from build123d import *

# Parameters (mm, degrees)
SKETCH1_W           = 47
SKETCH1_H           = 38.8
SKETCH1_R           = 2.5
SKETCH1_R_2         = 2.627
BOSS_EXTRUDE1_DEPTH = 106.999989
SKETCH2_R           = 3.571875
SKETCH2_R_2         = 4.92125
CUT_EXTRUDE1_DEPTH  = 39.8
SKETCH1_8_R         = 2.627
SKETCH1_8_R_2       = 2.5
CUT_EXTRUDE2_DEPTH  = 38.1
CUT_EXTRUDE3_START  = -47
SKETCH3_R           = 2
CUT_EXTRUDE3_DEPTH  = 25.4
SKETCH4_R           = 9.525
CUT_EXTRUDE4_DEPTH  = 21.0185


with BuildPart() as part:
    # Sketch1 → Boss-Extrude1 (new body)
    with BuildSketch(Plane(origin=(0, 0, 0), x_dir=(1, 0, 0), z_dir=(0, 1, 0))):
        with Locations((23.5, 19.4)):
            Rectangle(SKETCH1_W, SKETCH1_H)
        with Locations((4.5, 4.4)):
            Circle(SKETCH1_R, mode=Mode.SUBTRACT)
        with Locations((42.5, 4.4)):
            Circle(SKETCH1_R, mode=Mode.SUBTRACT)
        with Locations((4.5, 34.4)):
            Circle(SKETCH1_R_2, mode=Mode.SUBTRACT)
        with Locations((42.5, 34.4)):
            Circle(SKETCH1_R, mode=Mode.SUBTRACT)
        with Locations((42.5, 4.4)):
            Circle(SKETCH1_R)
        with Locations((4.5, 4.4)):
            Circle(SKETCH1_R)
        with Locations((4.5, 34.4)):
            Circle(SKETCH1_R_2)
        with Locations((42.5, 34.4)):
            Circle(SKETCH1_R)
    extrude(amount=BOSS_EXTRUDE1_DEPTH)

    # Sketch2 → Cut-Extrude1 (cut, through all)
    with BuildSketch(Plane.XY):
        with Locations((12.36448241, 63.94291018)):
            Circle(SKETCH2_R)
        with Locations((34.63551759, 63.94291018)):
            Circle(SKETCH2_R)
        with Locations((34.63551759, 41.671875)):
            Circle(SKETCH2_R)
        with Locations((23.5, 52.80739259)):
            Circle(SKETCH2_R_2)
        with Locations((12.36448241, 41.671875)):
            Circle(SKETCH2_R)
    extrude(amount=-CUT_EXTRUDE1_DEPTH, mode=Mode.SUBTRACT)

    # Sketch1<8> → Cut-Extrude2 (cut)
    with BuildSketch(Plane(origin=(0, 0, 0), x_dir=(1, 0, 0), z_dir=(0, 1, 0))):
        with Locations((4.5, 34.4)):
            Circle(SKETCH1_8_R)
        with Locations((4.5, 4.4)):
            Circle(SKETCH1_8_R_2)
        with Locations((42.5, 4.4)):
            Circle(SKETCH1_8_R_2)
        with Locations((42.5, 34.4)):
            Circle(SKETCH1_8_R_2)
    extrude(amount=CUT_EXTRUDE2_DEPTH, mode=Mode.SUBTRACT)

    # Sketch3 → Cut-Extrude3 (cut)
    with BuildSketch(Plane(origin=(47, 0, 0), x_dir=(0, 0, -1), z_dir=(1, 0, 0)).offset(CUT_EXTRUDE3_START)):
        with Locations((19.4, 20)):
            Circle(SKETCH3_R)
        with Locations((19.4, 79.944)):
            Circle(SKETCH3_R)
    extrude(amount=CUT_EXTRUDE3_DEPTH, mode=Mode.SUBTRACT)

    # Sketch4 → Cut-Extrude4 (cut)
    with BuildSketch(Plane(origin=(0, 0, -38.8), x_dir=(-1, 0, 0), z_dir=(0, 0, -1))):
        with Locations((-23.5, 52.80739259)):
            Circle(SKETCH4_R)
    extrude(amount=-CUT_EXTRUDE4_DEPTH, mode=Mode.SUBTRACT)


solid = part.part
Verification items for the finished model (mm, model axes). A direction names the side the tool comes from. Coordinates: 2 decimals unless noted, no trailing zeros. Order: outer loops, then holes, each group sorted by start corner. A loop starts at its lowest first (then second) coordinate and runs counter-clockwise, first axis right, second up. Notation, with made-up numbers: (-22, 64) -> (-5, 64) arc R6 ccw to (-5, 68) -> close; hole circle Ø1 at (7.5, 55). An arc over 180 degrees is marked (long way). Put each result on its own line as item: value. Start each with the question number.
1. Cross-section at A-A, the plane x = 23.5. Record the boundary of the cut face in (y, z), then the cut area to 3 significant figures.
2. Cross-section at B-B, the plane y = 20. Record the boundary of the cut face in (x, z), then the cut area to 3 significant figures.
3. Access from +Z, -Z, +X, -X, +Y, -Y to the whole of each face (thin tool, end or side, straight path). Record for faces 1 (the flat face through (4, 38.1, -34)), 2 (the cylindrical face through (11.59, 60.456, -19.128)), 3 (the flat face through (25.4, 20, -19)).
4. Cross-section at C-C, the plane x = 12.5. Record the boundary of the cut face in (y, z), then the cut area to 3 significant figures.
5. Material ranges on L1, parallel to X at y = 13.5, z = -4.5; L2, parallel to Z at x = 42.5, y = 8.5; L3, parallel to X at y = 29, z = -34.4, recorded low to high. Write a range as [from, to].
6. Go/stop test with flat-tipped pins: pin 1 Ø15 at (x, y) = (23.5, 51) entering from -Z; pin 2 Ø4 at (x, z) = (4.5, -4.4) entering from -Y. Record where each tip stops, or that it passes through.
7. Cross-section at D-D, the plane z = -25. Record the boundary of the cut face in (x, y) (3 decimals), then the cut area to 3 significant figures.
8. Mould release check, pull along Z, two halves, no side actions. Record for faces 4 (the flat face through (18, 53, 0)), 5 (the flat face through (19, 49, -17.781)), 6 (the cylindrical face through (12.522, 20.601, -21.308)): released by +Z, released by -Z, zero draft, split by the parting line, or undercut.
Computed:
1. outline: (0, -38.8) -> (43.28, -38.8) -> (43.28, -17.78) -> (47.89, -17.78) -> (47.89, 0) -> (0, 0) -> close; (57.73, -17.78) -> (62.33, -17.78) -> (62.33, -38.8) -> (107, -38.8) -> (107, 0) -> (57.73, 0) -> close; hole circle Ø4 at (20, -19.4); hole circle Ø4 at (79.94, -19.4)
1. area: 3,550 mm2
2. outline: (0, -38.8) -> (47, -38.8) -> (47, 0) -> (0, 0) -> (0, -17.4) -> (25.4, -17.4) -> (25.4, -21.4) -> (0, -21.4) -> close; hole circle Ø5.25 at (4.5, -34.4); hole circle Ø5 at (4.5, -4.4); hole circle Ø5 at (42.5, -34.4); hole circle Ø5 at (42.5, -4.4)
2. area: 1,640 mm2
3. face 1: -Y
3. face 2: +Z, -Z
3. face 3: -X
4. outline: (0, -38.8) -> (38.1, -38.8) -> (38.1, 0) -> (0, 0) -> close; (45.24, -38.8) -> (60.37, -38.8) -> (60.37, 0) -> (45.24, 0) -> close; (67.51, -38.8) -> (107, -38.8) -> (107, 0) -> (67.51, 0) -> close; hole circle Ø4 at (20, -19.4); hole circle Ø4 at (79.94, -19.4)
4. area: 3,570 mm2
5. L1: [0, 2], [7, 40], [45, 47]
5. L2: [-38.8, -36.9], [-31.9, -6.9], [-1.9, 0]
5. L3: [0, 1.87], [7.13, 40], [45, 47]
6. pin 1: z = -17.78
6. pin 2: y = 38.1
7. outline: (0, 0) -> (47, 0) -> (47, 107) -> (0, 107) -> close; hole circle Ø7.144 at (12.364, 41.672); hole circle Ø7.144 at (12.364, 63.943); hole circle Ø19.05 at (23.5, 52.807); hole circle Ø7.144 at (34.636, 41.672); hole circle Ø7.144 at (34.636, 63.943)
7. area: 4,580 mm2
8. face 4: released by +Z
8. face 5: released by -Z
8. face 6: undercut
